from build123d import *

# Parameters (mm, degrees)
F0_R     = 1.45
F0_W     = 10
F0_H     = 3
F0_W_2   = 3
F0_H_2   = 10
F1_DEPTH = 3
F2_R     = 1.65
F2_W     = 2.98
F2_H     = 5
F2_W_2   = 39.9
F2_H_2   = 19.4
F3_DEPTH = 25
F2_R_2   = 1.45
F4_DEPTH = 3
F5_W     = 10
F5_H     = 2.98
F6_DEPTH = 12.5


with BuildPart() as f1:
    # F0 (on Right) → F1 (new body)
    with BuildSketch(Plane.YZ):
        Polygon((-35, 50), (-50, 50), (-50, 35), (-47, 35), (-47, 25), (-50, 25), (-50, 5), (-47, 5), (-47, -5), (-50, -5), (-50, -25), (-47, -25), (-47, -35), (-50, -35), (-50, -50), (-35, -50), (-35, -47), (-25, -47), (-25, -50), (-5, -50), (-5, -47), (5, -47), (5, -50), (25, -50), (25, -47), (35, -47), (35, -50), (50, -50), (50, -35), (47, -35), (47, -25), (50, -25), (50, -5), (47, -5), (47, 5), (50, 5), (50, 25), (47, 25), (47, 35), (50, 35), (50, 50), (35, 50), (35, 47), (25, 47), (25, 50), (5, 50), (5, 47), (-5, 47), (-5, 50), (-25, 50), (-25, 47), (-35, 47), align=None)
        with Locations((-8, -20)):
            Circle(F0_R, mode=Mode.SUBTRACT)
        with Locations((-30, 51.5)):
            Rectangle(F0_W, F0_H)
        with Locations((-30, 48.5)):
            Rectangle(F0_W, F0_H)
        with Locations((-48.5, 30)):
            Rectangle(F0_W_2, F0_H_2)
        with Locations((-51.5, 30)):
            Rectangle(F0_W_2, F0_H_2)
        with Locations((0, 51.5)):
            Rectangle(F0_W, F0_H)
        with Locations((0, 48.5)):
            Rectangle(F0_W, F0_H)
        with Locations((-48.5, 0)):
            Rectangle(F0_W_2, F0_H_2)
        with Locations((-51.5, 0)):
            Rectangle(F0_W_2, F0_H_2)
        with Locations((30, 51.5)):
            Rectangle(F0_W, F0_H)
        with Locations((30, 48.5)):
            Rectangle(F0_W, F0_H)
        with Locations((-48.5, -30)):
            Rectangle(F0_W_2, F0_H_2)
        with Locations((-51.5, -30)):
            Rectangle(F0_W_2, F0_H_2)
        with Locations((51.5, 30)):
            Rectangle(F0_W_2, F0_H_2)
        with Locations((48.5, 30)):
            Rectangle(F0_W_2, F0_H_2)
        with Locations((-30, -48.5)):
            Rectangle(F0_W, F0_H)
        with Locations((-30, -51.5)):
            Rectangle(F0_W, F0_H)
        with Locations((51.5, 0)):
            Rectangle(F0_W_2, F0_H_2)
        with Locations((48.5, 0)):
            Rectangle(F0_W_2, F0_H_2)
        with Locations((0, -48.5)):
            Rectangle(F0_W, F0_H)
        with Locations((0, -51.5)):
            Rectangle(F0_W, F0_H)
        with Locations((51.5, -30)):
            Rectangle(F0_W_2, F0_H_2)
        with Locations((48.5, -30)):
            Rectangle(F0_W_2, F0_H_2)
        with Locations((30, -48.5)):
            Rectangle(F0_W, F0_H)
        with Locations((30, -51.5)):
            Rectangle(F0_W, F0_H)
    extrude(amount=F1_DEPTH)

    # F2 (on face) → F3 (cut)
    with BuildSketch(Plane(origin=(0, 0, 0), x_dir=(0, -1, 0), z_dir=(-1, 0, 0))):
        with Locations((-4.05, 29.7)):
            Circle(F2_R)
        with Locations((-4.05, 19.7)):
            Circle(F2_R)
        with Locations((43.95, 29.7)):
            Circle(F2_R)
        with Locations((43.95, 19.7)):
            Circle(F2_R)
        with Locations((11.4694618905, 9.5)):
            Rectangle(F2_W, F2_H)
        with Locations((28.4305381095, 9.5)):
            Rectangle(F2_W, F2_H)
        with Locations((19.95, 24.7)):
            Rectangle(F2_W_2, F2_H_2)
        with Locations((19.95, 39.9)):
            Rectangle(F2_W, F2_H)
    extrude(amount=-F3_DEPTH, mode=Mode.SUBTRACT)

    # F2 (on face) → F4 (join)
    with BuildSketch(Plane(origin=(0, 0, 0), x_dir=(0, -1, 0), z_dir=(-1, 0, 0))):
        Polygon((-50, 50), (-50, 35), (50, 35), (50, 50), (35, 50), (25, 50), (5, 50), (-5, 50), (-25, 50), (-35, 50), align=None)
        with Locations((19.95, 39.9)):
            Rectangle(F2_W, F2_H, mode=Mode.SUBTRACT)
        Polygon((-50, -35), (-50, -50), (-35, -50), (-25, -50), (-5, -50), (5, -50), (25, -50), (35, -50), (50, -50), (-20, 13), (-50, 13), (-50, 5), (-50, -5), (-50, -25), align=None)
        with Locations((8, -20)):
            Circle(F2_R_2, mode=Mode.SUBTRACT)
    extrude(amount=F4_DEPTH)

    # F5 (on Right) → F6 (cut, symmetric)
    with BuildSketch(Plane.YZ):
        with Locations((7, -45)):
            Rectangle(F5_W, F5_H)
        with Locations((-23, -45)):
            Rectangle(F5_W, F5_H)
        with Locations((-8, -35)):
            Rectangle(F5_W, F5_H)
    extrude(amount=F6_DEPTH, both=True, mode=Mode.SUBTRACT)


solid = f1.part
Source: CAD feature listing. Evaluate the final solid. Frame: model axes, mm. A direction names the side the tool comes from. Round coordinates to 2 decimals unless told otherwise and drop trailing zeros. Write each loop counter-clockwise with the first axis right and the second up, starting at its lowest first coordinate (ties: lowest second). Pieces come first, ordered by that corner, then holes. Notation, with made-up numbers: M 44,67.25 L 51,67.25 A18 cw 51,95.25 Z; hole C -27.75,-2.5 d4. An arc over 180 degrees is marked long. One line per item, written item: value. Start each with the question number.
Item 1: Pin query (flat end, axial travel): pin 1 (1.8 mm diameter, centred on x = -1, y = -21, fed in from +Z); pin 2 (2.5 mm diameter, centred on x = 1, z = 40.5, fed in from +Y); pin 3 (3.5 mm diameter, centred on x = 1, z = -51.5, fed in from -Y). Return the tip coordinate at first contact, or that it passes through.
Item 2: Ray query, L1, parallel to Z at x = 1.4, y = -43.95; L2, parallel to Z at x = 1.4, y = 4.05; L3, parallel to Z at x = 2.6, y = -24. Return the intervals inside material, ascending. Write a range as from..to.
Item 3: Section query C-C (y = -8). Return the cut outline in (x, z), plus the area to 3 significant figures.
Item 4: Set-up query: faces 1 (the flat face through (1, -20, 34.4)), 2 (the flat face through (1, -5, 51)), 3 (the flat face through (0, 30, 52)), 4 (the flat face through (1, -52, 5)), 5 (the flat face through (1, 51, 25)). Return all of +Z, -Z, +X, -X, +Y, -Y with unobstructed straight access to the full face (end or side cutting, diameter ignored); none if empty.
Item 5: Section query A-A (x = -1.25). Return the cut outline in (y, z), plus the area to 3 significant figures.
Item 6: Section query D-D (y = 29). Return the cut outline in (x, z).
Item 7: Section query B-B (z = 19.7). Return the cut outline in (x, y).
Item 8: Mould query, pull axis Y, two halves, no side actions, for faces 6 (the flat face through (1, -53, 30)), 7 (the flat face through (1, -30, -53)), 8 (the flat face through (-1, -1, -50)). Classes: pulls with the +Y half, pulls with the -Y half, needs draft (parallel to the pull), parting line crosses it, or undercut.
Result set:
1. pin 1: stops at z = 50
1. pin 2: stops at y = 50
1. pin 3: stops at y = -50
2. L1: z = -50..18.05, 21.35..28.05, 31.35..50
2. L2: z = -53..-46.49, -43.51..18.05, 21.35..28.05, 31.35..53
2. L3: z = -50..-46.49, -43.51..15, 34.4..50
3. outline: M -3,-50 L 3,-50 L 3,-36.49 L -3,-36.49 Z; M -3,-33.51 L 3,-33.51 L 3,-21.45 L -3,-21.45 Z; M -3,-18.55 L 3,-18.55 L 3,15 L 0,15 L 0,-12.2 L -3,-12.2 Z; M -3,35 L 0,35 L 0,34.4 L 3,34.4 L 3,50 L -3,50 Z
3. area: 365 mm²
4. face 1: +X, -X
4. face 2: +Z, +X, -X
4. face 3: +Z, -X, +Y, -Y
4. face 4: +X, -X, -Y
4. face 5: +X, -X, +Y
5. outline: M -50,-50 L 50,-50 L 50,13 L 20,13 Z; M -50,35 L 50,35 L 50,50 L -50,50 Z; hole M -28,-46.49 L -18,-46.49 L -18,-43.51 L -28,-43.51 Z; hole M -21.44,37.4 L -18.46,37.4 L -18.46,42.4 L -21.44,42.4 Z; hole M -13,-36.49 L -3,-36.49 L -3,-33.51 L -13,-33.51 Z; hole C -8,-20 d2.9; hole M 2,-46.49 L 12,-46.49 L 12,-43.51 L 2,-43.51 Z
5. area: 5,480 mm²
6. outline: M -3,-50 L 0,-50 L 0,-53 L 3,-53 L 3,53 L 0,53 L 0,50 L -3,50 L -3,35 L 0,35 L 0,13 L -3,13 Z
7. outline: M 0,-50 L 3,-50 L 3,-45.6 L 0,-45.6 Z; M 0,-42.3 L 3,-42.3 L 3,-39.9 L 0,-39.9 Z; M 0,0 L 3,0 L 3,2.4 L 0,2.4 Z; M 0,5.7 L 3,5.7 L 3,50 L 0,50 Z
8. face 6: pulls with the -Y half
8. face 7: needs draft
8. face 8: undercut
